```python
from build123d import *

# Parameters (mm, degrees)
ESBO_O1_W                = 31.2
ESBO_O1_H                = 13.9
RESSALTO_EXTRUS_O1_DEPTH = 1.58
ESBO_O2_W                = 7
ESBO_O2_H                = 6.9
ESBO_O2_H_2              = 0.1
RESSALTO_EXTRUS_O2_DEPTH = 5
RESSALTO_EXTRUS_O3_DEPTH = 10.5
CHANFRO1_SIZE            = 0.5
ESBO_O4_W                = 2.5
ESBO_O4_H                = 9.457135355
RESSALTO_EXTRUS_O4_DEPTH = 2.65
ESBO_O5_W                = 0.65
ESBO_O5_H                = 0.65
RESSALTO_EXTRUS_O5_DEPTH = 8.25
PADR_O_LINEAR1_COUNT     = 4
PADR_O_LINEAR1_PITCH     = 2


with BuildPart() as part:
    # Esboço1 → Ressalto-extrusão1 (new body)
    with BuildSketch(Plane(origin=(0, 0, 0), x_dir=(1, 0, 0), z_dir=(0, 1, 0))):
        Rectangle(ESBO_O1_W, ESBO_O1_H)
    extrude(amount=RESSALTO_EXTRUS_O1_DEPTH)

    # Esboço2 → Ressalto-extrusão2 (add)
    with BuildSketch(Plane(origin=(0, 1.58, 0), x_dir=(1, 0, 0), z_dir=(0, 1, 0))):
        with Locations((1.086462839, -3.5)):
            Rectangle(ESBO_O2_W, ESBO_O2_H)
        with Locations((1.086462839, -7)):
            Rectangle(ESBO_O2_W, ESBO_O2_H_2)
    extrude(amount=RESSALTO_EXTRUS_O2_DEPTH)

    # Esboço3 → Ressalto-extrusão3 (add)
    with BuildSketch(Plane.XZ):
        Polygon((12.918626435, -5.363327787), (14.320868257, -3.961085964), (14.320868257, 4.636672213), (8.820868257, 4.636672213), (8.820868257, -3.961085964), (9.855714298, -5.363327787), align=None)
    extrude(amount=RESSALTO_EXTRUS_O3_DEPTH)

    # Chanfro1
    chanfro1_edges = [part.edges().sort_by_distance(p)[0] for p in [
        (11.570868257, -10.5, 4.636672213),
        (8.820868257, -10.5, 0.337793125),
        (9.338291278, -10.5, -4.662206875),
        (11.387170366, -10.5, -5.363327787),
        (13.619747346, -10.5, -4.662206875),
        (14.320868257, -10.5, 0.337793125),
    ]]
    chamfer(chanfro1_edges, length=CHANFRO1_SIZE)

    # Esboço4 → Ressalto-extrusão4 (add)
    with BuildSketch(Plane(origin=(0, 1.58, 0), x_dir=(1, 0, 0), z_dir=(0, 1, 0))):
        with Locations((-13.088241827, -0.331483756)):
            Rectangle(ESBO_O4_W, ESBO_O4_H)
    extrude(amount=RESSALTO_EXTRUS_O4_DEPTH)

    # Esboço5 → Ressalto-extrusão5 (add)
    with BuildSketch(Plane(origin=(0, 4.23, 0), x_dir=(1, 0, 0), z_dir=(0, 1, 0))):
        with Locations((-13.025924603, 3.050020292)):
            Rectangle(ESBO_O5_W, ESBO_O5_H)
    ressalto_extrus_o5 = extrude(amount=RESSALTO_EXTRUS_O5_DEPTH)

    # Padrão linear1: Ressalto-extrusão5 ×4
    with Locations(*[(0, 0, i * PADR_O_LINEAR1_PITCH) for i in range(1, PADR_O_LINEAR1_COUNT)]):
        add(ressalto_extrus_o5)


solid = part.part
```
Design review of the part built by this model. Coordinates are the model's own, in mm. A direction names the side the tool comes from. Round coordinates to 2 decimals unless told otherwise and drop trailing zeros. Write each loop counter-clockwise with the first axis right and the second up, starting at its lowest first coordinate (ties: lowest second). Pieces come first, ordered by that corner, then holes. Notation, with made-up numbers: (0.25, 4) -> (15.25, 4) arc R24 cw to (15.25, 20) -> close; hole circle Ø11 at (-30, 34). An arc over 180 degrees is marked (long way). Write item = value, one per line. Start each with the question number.
1) Tool access review of faces 1 (the face through (1, 4, 0.05)), 2 (the face through (11, -5, -5.363)), 3 (the face through (9.33, -4.93, -4.65)), 4 (the face through (0, 1, 6.95)), 5 (the face through (14.321, -5, 0)): name each direction out of +Z, -Z, +X, -X, +Y, -Y from which nothing blocks a thin tool from reaching the whole face with its end or side.
2) Clearance check with flat-ended pins moving along their axes: pin 1 (1.5 mm diameter, centred on x = 6.5, z = -4, fed in from -Y); pin 2 (7 mm diameter, centred on x = -6.5, z = -2.5, fed in from +Y); pin 3 (3 mm diameter, centred on x = 10.5, y = -3, fed in from +Z). State where each tip first meets the part, or that it passes through.
3) Take a section at A-A, the plane y = 6. State the section outline as (x, z) points, plus the area to 3 significant figures.
4) Wall thickness on probe 1 along X at (y, z) = (2.75, 4); probe 2 along Y at (x, z) = (-5.5, 1.5); probe 3 along Z at (x, y) = (-13, 2.5): over which ranges is each line inside the solid? List them lowest first. Write a range as from..to.
5) Mouldability with a two-part tool opening along X and no side actions: class faces 6 (the face through (-13, 3, 5.06)), 7 (the face through (8.821, -5, 0)), 8 (the face through (-2.414, 4, 4)), 9 (the face through (-11.838, 3, 0)) as +X half, -X half, draft (parallel to the pull), parting line (faces both ways), or undercut.
6) Take a section at D-D, the plane y = -5.25. State the section outline as (x, z) points.
7) Take a section at C-C, the plane z = 6.25. State the section outline as (x, y) points.
8) Take a section at B-B, the plane x = 3. State the section outline as (y, z) points.
Results list:
q1.face_1 = -Z, +X, +Y
q1.face_2 = -Z, +X, -X, -Y
q1.face_3 = -Z, -X, -Y
q1.face_4 = +Z, +X, -X, -Y
q1.face_5 = +Z, -Z, +X, -Y
q2.pin_1 = 0
q2.pin_2 = 1.58
q2.pin_3 = 4.64
q3.outline = (-13.35, -3.38) -> (-12.7, -3.38) -> (-12.7, -2.73) -> (-13.35, -2.73) -> close; (-13.35, -1.38) -> (-12.7, -1.38) -> (-12.7, -0.73) -> (-13.35, -0.73) -> close; (-13.35, 0.62) -> (-12.7, 0.62) -> (-12.7, 1.27) -> (-13.35, 1.27) -> close; (-13.35, 2.62) -> (-12.7, 2.62) -> (-12.7, 3.27) -> (-13.35, 3.27) -> close; (-2.41, 0.05) -> (4.59, 0.05) -> (4.59, 7.05) -> (-2.41, 7.05) -> close
q3.area = 50.7 mm²
q4.probe_1 = -14.34..-11.84, -2.41..4.59
q4.probe_2 = 0..1.58
q4.probe_3 = -4.4..5.06
q5.face_6 = draft
q5.face_7 = -X half
q5.face_8 = undercut
q5.face_9 = undercut
q6.outline = (8.82, -3.96) -> (9.86, -5.36) -> (12.92, -5.36) -> (14.32, -3.96) -> (14.32, 4.64) -> (8.82, 4.64) -> close
q7.outline = (-15.6, 0) -> (15.6, 0) -> (15.6, 1.58) -> (4.59, 1.58) -> (4.59, 6.58) -> (-2.41, 6.58) -> (-2.41, 1.58) -> (-15.6, 1.58) -> close
q8.outline = (0, -6.95) -> (1.58, -6.95) -> (1.58, 0.05) -> (6.58, 0.05) -> (6.58, 7.05) -> (1.58, 7.05) -> (1.58, 6.95) -> (0, 6.95) -> close
